Autodesk Inventor part; units mm, degrees
ref_plane "BODY_N_XY" through (247, 0, 0) normal (0, 0, -1) x (1, 0, 0)
ref_plane "BODY_N_YZ" through (247, 0, 0) normal (1, 0, 0) x (0, -1, 0)
ref_plane "BODY_N_ZX" through (247, 0, 0) normal (0, -1, 0) x (0, 0, -1)
sketch "Sketch_8" plane through (0, 0, 0) normal (0, 0, 1) x (1, 0, 0)
  line L0 (0, 0) -> (-8, 0)
  line L1 (-8, 0) -> (-8, 4.3865)
  line L2 (-8, 4.3865) -> (-7.3865, 5)
  line L3 (-7.3865, 5) -> (0, 5)
  line L4 (0, 5) -> (0, 0)
  line L5 (0, 0) -> (-8, 0)
revolve "Revolution1" add sketch "Sketch_8" angle 360 about axis through (0, 0, 0) along (1, 0, 0)
thread "Thread1"
sketch "Sketch_9" plane through (0, 0, 0) normal (1, 0, 0) x (0, 0, -1)
  line L0 (-9.15, 4.0345) -> (-9.15, -4.0345)
  arc A0 (-9.15, -4.0345) -> (-4.0345, -9.15) centre (0, 0) ccw
  line L1 (-4.0345, -9.15) -> (4.0345, -9.15)
  arc A1 (4.0345, -9.15) -> (9.15, -4.0345) centre (0, 0) ccw
  line L2 (9.15, -4.0345) -> (9.15, 4.0345)
  arc A2 (9.15, 4.0345) -> (4.0345, 9.15) centre (0, 0) ccw
  line L3 (4.0345, 9.15) -> (-4.0345, 9.15)
  arc A3 (-4.0345, 9.15) -> (-9.15, 4.0345) centre (0, 0) ccw
extrude "Extrusion1" add sketch "Sketch_9" along normal blind 12.5
sketch "Sketch_11" plane through (12.5, 0, 0) normal (1, 0, 0) x (0, 0, -1)
  circle A0 centre (0, 0) radius 8.7
extrude "Extrusion2" add sketch "Sketch_11" along normal blind 225
sketch "Sketch_10" plane through (237.5, 0, 0) normal (1, 0, 0) x (0, 0, -1)
  line L0 (-9.15, 4.0345) -> (-9.15, -4.0345)
  arc A0 (-9.15, -4.0345) -> (-4.0345, -9.15) centre (0, 0) ccw
  line L1 (-4.0345, -9.15) -> (4.0345, -9.15)
  arc A1 (4.0345, -9.15) -> (9.15, -4.0345) centre (0, 0) ccw
  line L2 (9.15, -4.0345) -> (9.15, 4.0345)
  arc A2 (9.15, 4.0345) -> (4.0345, 9.15) centre (0, 0) ccw
  line L3 (4.0345, 9.15) -> (-4.0345, 9.15)
  arc A3 (-4.0345, 9.15) -> (-9.15, 4.0345) centre (0, 0) ccw
extrude "Extrusion3" add sketch "Sketch_10" along normal blind 9.5
sketch "Sketch7" plane through (0, 0, 0) normal (0, 0, 1) x (1, 0, 0)
  line L0 (8, 9.15) -> (8, 4.15)
  line L1 (8, 2.9566) -> (5.933, 4.15)
  line L2 (5.933, 4.15) -> (5.933, 8.717)
  line L3 (5.933, 8.717) -> (5.5, 9.15)
  line L4 (5.5, 9.15) -> (8, 9.15)
  line L5 (8, 9.15) -> (8, 2.9566)
revolve "Revolution2" cut sketch "Sketch7" angle 360 about axis through (8, 9.15, 0) along (0, 1, 0)
thread "Thread2"
sketch "Sketch_7" plane through (0, 0, 0) normal (0, 0, 1) x (1, 0, 0)
  line L0 (242, 9.15) -> (242, 4.15)
  line L1 (242, 2.9566) -> (239.933, 4.15)
  line L2 (239.933, 4.15) -> (239.933, 8.717)
  line L3 (239.933, 8.717) -> (239.5, 9.15)
  line L4 (239.5, 9.15) -> (242, 9.15)
  line L5 (242, 9.15) -> (242, 2.9566)
revolve "Revolution3" cut sketch "Sketch_7" angle 360 about axis through (242, 9.15, 0) along (0, 1, 0)
thread "Thread3"
sketch "Sketch_16" plane through (0, 0, 0) normal (0, 0, 1) x (1, 0, 0)
  line L0 (217.5, 0) -> (-8, 0)
  line L1 (-8, 0) -> (-8, 2.5)
  line L2 (-8, 2.5) -> (12.5, 2.5)
  line L3 (12.5, 2.5) -> (12.5, 8)
  line L4 (12.5, 8) -> (217.5, 8)
  line L5 (217.5, 8) -> (217.5, 0)
  line L6 (217.5, 0) -> (-8, 0)
revolve "Revolution4" cut sketch "Sketch_16" angle 360 about axis through (217.5, 0, 0) along (1, 0, 0)
ref_plane "BODY_N_XY" through (247, 0, 0) normal (0, 0, -1) x (1, 0, 0)
ref_plane "BODY_N_YZ" through (247, 0, 0) normal (1, 0, 0) x (0, -1, 0)
ref_plane "BODY_N_ZX" through (247, 0, 0) normal (0, -1, 0) x (0, 0, -1)
ref_plane "NUT2_XY" through (247, 0, 0) normal (1, 0, 0) x (0, 0, -1)
ref_plane "NUT2_YZ" through (247, 0, 0) normal (0, 0, -1) x (0, 1, 0)
ref_plane "NUT2_ZX" through (247, 0, 0) normal (0, 1, 0) x (1, 0, 0)
ref_plane "SW1_XY" through (17.5, 0, 0) normal (1, 0, 0) x (0, 0, -1)
ref_plane "SW1_YZ" through (17.5, 0, 0) normal (0, 0, -1) x (0, 1, 0)
ref_plane "SW1_ZX" through (17.5, 0, 0) normal (0, 1, 0) x (1, 0, 0)
ref_plane "SW2_XY" through (232.5, 0, 0) normal (-1, 0, 0) x (0, 0, -1)
ref_plane "SW2_YZ" through (232.5, 0, 0) normal (0, 0, -1) x (0, -1, 0)
ref_plane "SW2_ZX" through (232.5, 0, 0) normal (0, -1, 0) x (-1, 0, 0)
ref_plane "SW_R1_XY" through (17.5, -14.15, 0) normal (1, 0, 0) x (0, 0, -1)
ref_plane "SW_R1_YZ" through (17.5, -14.15, 0) normal (0, 0, -1) x (0, 1, 0)
ref_plane "SW_R1_ZX" through (17.5, -14.15, 0) normal (0, 1, 0) x (1, 0, 0)
ref_plane "SW_R2_XY" through (232.5, -14.15, 0) normal (-1, 0, 0) x (0, 0, -1)
ref_plane "SW_R2_YZ" through (232.5, -14.15, 0) normal (0, 0, -1) x (0, -1, 0)
ref_plane "SW_R2_ZX" through (232.5, -14.15, 0) normal (0, -1, 0) x (-1, 0, 0)
ref_plane "body_XY" through (0, 0, 0) normal (1, 0, 0) x (0, 0, -1)
ref_plane "body_YZ" through (0, 0, 0) normal (0, 0, -1) x (0, 1, 0)
ref_plane "body_ZX" through (0, 0, 0) normal (0, 1, 0) x (1, 0, 0)
properties part number "CJ2B16-200Z(1_0)_BODY" material "鉄、鋳鉄"
Geometry check sheet. Reference: the model listing, model coordinates, mm. A direction names the side the tool comes from. Coordinates: 2 decimals unless noted, no trailing zeros. Loops run counter-clockwise (first coordinate to the right, second up) from the corner with the lowest first, then second, coordinate; pieces in that order, holes last. Notation, with made-up numbers: (88.25, 6.25) - (135.25, 6.25) arc R14 ccw to (135.25, 16.25) - close; hole circle Ø9 at (18, 39). An arc over 180 degrees is marked (long way). One line per item, written item: value. Start each with the question number.
(1) Mould release check, pull along X, two halves, no side actions. Record for faces 4 (the flat face through (12.5, -9, 1)), 5 (the flat face through (0, -4, -4)), 6 (the cylindrical face through (242.18, 7.11, -7.03)), 7 (the conical face through (242.28, 3.16, -0.22)): released by +X, released by -X, zero draft, split by the parting line, or undercut.
(2) Tool access check on faces 1 (the flat face through (217.5, 0, 0)), 2 (the flat face through (6, 0, -9.15)), 3 (the cylindrical face through (244.065, 6.465, 0.091)). Record the directions out of +Z, -Z, +X, -X, +Y, -Y that give a thin tool (end or side, any length) a straight path to the whole face; none if there is none.
(3) Depth check by flat-ended pin: P1, Ø5, axis at y = -4, z = -2, coming from the -X side; P2, Ø4, axis at x = 175, y = 1, coming from the +Z side; P3, Ø6, axis at x = 49.5, y = -5.5, coming from the +Z side; P4, Ø1.5, axis at x = 112.5, z = -1.5, coming from the -Y side. Enter the tip coordinate at first touch or a pass-through.
(4) Cross-section at A-A on x = 129. Enter the section's corners in (y, z), plus the area to 3 significant figures.
(5) Material ranges on line 1 (X direction, y = 6, z = 4.25); line 2 (Z direction, x = -2.5, y = 0); line 3 (X direction, y = -8, z = 1), recorded low to high. Write a range as [from, to].
Results below:
1. face 4: undercut
1. face 5: released by -X
1. face 6: zero draft
1. face 7: undercut
2. face 1: none
2. face 2: -Z, +X, -X, +Y, -Y
2. face 3: +Y
3. P1: stops at x = -8
3. P2: stops at z = 8.7
3. P3: stops at z = 8.33
3. P4: stops at y = -8.67
4. outline: circle Ø17.4 at (0, 0); hole circle Ø16 at (0, 0)
4. area: 36.7 mm2
5. line 1: x = [0, 12.5], [217.5, 247]
5. line 2: z = [-5, -2.5], [2.5, 5]
5. line 3: x = [0, 247]
